from build123d import *

# Parameters (mm, degrees)
SKETCH2_R           = 2.75
BOSS_EXTRUDE1_DEPTH = 60
BOSS_EXTRUDE2_DEPTH = 2


with BuildPart() as part:
    # Sketch2 → Boss-Extrude1 (new body)
    with BuildSketch(Plane(origin=(0, 0, 0), x_dir=(1, 0, 0), z_dir=(0, 1, 0))):
        with BuildLine():
            Line((87, -11), (87, 88))
            ThreePointArc((87, 88), (84.656854249, 93.656854249), (79, 96))
            Line((79, 96), (39, 96))
            ThreePointArc((39, 96), (36.171572875, 94.828427125), (35, 92))
            Line((35, 92), (35, 44))
            ThreePointArc((35, 44), (33.828427125, 41.171572875), (31, 40))
            Line((31, 40), (-31, 40))
            ThreePointArc((-31, 40), (-33.828427125, 41.171572875), (-35, 44))
            Line((-35, 44), (-35, 92))
            ThreePointArc((-35, 92), (-36.171572875, 94.828427125), (-39, 96))
            Line((-39, 96), (-79, 96))
            ThreePointArc((-79, 96), (-84.656854249, 93.656854249), (-87, 88))
            Line((-87, 88), (-87, -11))
            ThreePointArc((-87, -11), (-84.656854249, -16.656854249), (-79, -19))
            Line((-79, -19), (-32, -19))
            ThreePointArc((-32, -19), (-29.171572875, -17.828427125), (-28, -15))
            Line((-28, -15), (-28, -3))
            ThreePointArc((-28, -3), (0, 25), (28, -3))
            Line((28, -3), (28, -15))
            ThreePointArc((28, -15), (29.171572875, -17.828427125), (32, -19))
            Line((32, -19), (79, -19))
            ThreePointArc((79, -19), (84.656854249, -16.656854249), (87, -11))
        make_face()
        with Locations(Location((-79, 88, 0), (0, 0, 270))):
            Circle(SKETCH2_R, mode=Mode.SUBTRACT)
        with Locations(Location((79, 88, 0), (0, 0, 270))):
            Circle(SKETCH2_R, mode=Mode.SUBTRACT)
        with Locations(Location((79, -11, 0), (0, 0, 270))):
            Circle(SKETCH2_R, mode=Mode.SUBTRACT)
        with Locations(Location((-79, -11, 0), (0, 0, 270))):
            Circle(SKETCH2_R, mode=Mode.SUBTRACT)
        with Locations(Location((0, 32.5, 0), (0, 0, 270))):
            Circle(SKETCH2_R, mode=Mode.SUBTRACT)
        with BuildLine():
            Line((-39, 93.5), (-71.5, 93.5))
            ThreePointArc((-71.5, 93.5), (-72.914213562, 92.914213562), (-73.5, 91.5))
            Line((-73.5, 91.5), (-73.5, 88))
            ThreePointArc((-73.5, 88), (-75.110912703, 84.110912703), (-79, 82.5))
            Line((-79, 82.5), (-82.5, 82.5))
            ThreePointArc((-82.5, 82.5), (-83.914213562, 81.914213562), (-84.5, 80.5))
            Line((-84.5, 80.5), (-84.5, -3.5))
            ThreePointArc((-84.5, -3.5), (-83.914213562, -4.914213562), (-82.5, -5.5))
            Line((-82.5, -5.5), (-79, -5.5))
            ThreePointArc((-79, -5.5), (-75.110912703, -7.110912703), (-73.5, -11))
            Line((-73.5, -11), (-73.5, -14.5))
            ThreePointArc((-73.5, -14.5), (-72.914213562, -15.914213562), (-71.5, -16.5))
            Line((-71.5, -16.5), (-32, -16.5))
            ThreePointArc((-32, -16.5), (-30.939339828, -16.060660172), (-30.5, -15))
            Line((-30.5, -15), (-30.5, -3))
            ThreePointArc((-30.5, -3), (-23.549354883, 16.382411734), (-5.865384615, 26.930707698))
            ThreePointArc((-5.865384615, 26.930707698), (-4.705780008, 27.622399237), (-4.25, 28.893377055))
            Line((-4.25, 28.893377055), (-4.25, 35.5))
            ThreePointArc((-4.25, 35.5), (-4.835786438, 36.914213562), (-6.25, 37.5))
            Line((-6.25, 37.5), (-31, 37.5))
            ThreePointArc((-31, 37.5), (-35.596194078, 39.403805922), (-37.5, 44))
            Line((-37.5, 44), (-37.5, 92))
            ThreePointArc((-37.5, 92), (-37.939339828, 93.060660172), (-39, 93.5))
        make_face(mode=Mode.SUBTRACT)
        with BuildLine():
            Line((30.5, -15), (30.5, -3))
            ThreePointArc((30.5, -3), (23.549354883, 16.382411734), (5.865384615, 26.930707698))
            ThreePointArc((5.865384615, 26.930707698), (4.705780008, 27.622399237), (4.25, 28.893377055))
            Line((4.25, 28.893377055), (4.25, 35.5))
            ThreePointArc((4.25, 35.5), (4.835786438, 36.914213562), (6.25, 37.5))
            Line((6.25, 37.5), (31, 37.5))
            ThreePointArc((31, 37.5), (35.596194078, 39.403805922), (37.5, 44))
            Line((37.5, 44), (37.5, 92))
            ThreePointArc((37.5, 92), (37.939339828, 93.060660172), (39, 93.5))
            Line((39, 93.5), (71.5, 93.5))
            ThreePointArc((71.5, 93.5), (72.914213562, 92.914213562), (73.5, 91.5))
            Line((73.5, 91.5), (73.5, 88))
            ThreePointArc((73.5, 88), (75.110912703, 84.110912703), (79, 82.5))
            Line((79, 82.5), (82.5, 82.5))
            ThreePointArc((82.5, 82.5), (83.914213562, 81.914213562), (84.5, 80.5))
            Line((84.5, 80.5), (84.5, -3.5))
            ThreePointArc((84.5, -3.5), (83.914213562, -4.914213562), (82.5, -5.5))
            Line((82.5, -5.5), (79, -5.5))
            ThreePointArc((79, -5.5), (75.110912703, -7.110912703), (73.5, -11))
            Line((73.5, -11), (73.5, -14.5))
            ThreePointArc((73.5, -14.5), (72.914213562, -15.914213562), (71.5, -16.5))
            Line((71.5, -16.5), (32, -16.5))
            ThreePointArc((32, -16.5), (30.939339828, -16.060660172), (30.5, -15))
        make_face(mode=Mode.SUBTRACT)
    extrude(amount=BOSS_EXTRUDE1_DEPTH)

    # Sketch3 → Boss-Extrude2 (add)
    # profile 1 of 2: a face of its own
    with BuildSketch(Plane.XZ):
        with BuildLine():
            Line((-37.5, -92), (-37.5, -44))
            ThreePointArc((-37.5, -44), (-35.596194078, -39.403805922), (-31, -37.5))
            Line((-31, -37.5), (-6.25, -37.5))
            ThreePointArc((-6.25, -37.5), (-4.835786438, -36.914213562), (-4.25, -35.5))
            Line((-4.25, -35.5), (-4.25, -28.893377055))
            ThreePointArc((-4.25, -28.893377055), (-4.705780008, -27.622399237), (-5.865384615, -26.930707698))
            ThreePointArc((-5.865384615, -26.930707698), (-23.549354883, -16.382411734), (-30.5, 3))
            Line((-30.5, 3), (-30.5, 15))
            ThreePointArc((-30.5, 15), (-30.939339828, 16.060660172), (-32, 16.5))
            Line((-32, 16.5), (-71.5, 16.5))
            ThreePointArc((-71.5, 16.5), (-72.914213562, 15.914213562), (-73.5, 14.5))
            Line((-73.5, 14.5), (-73.5, 11))
            ThreePointArc((-73.5, 11), (-75.110912703, 7.110912703), (-79, 5.5))
            Line((-79, 5.5), (-82.5, 5.5))
            ThreePointArc((-82.5, 5.5), (-83.914213562, 4.914213562), (-84.5, 3.5))
            Line((-84.5, 3.5), (-84.5, -80.5))
            ThreePointArc((-84.5, -80.5), (-83.914213562, -81.914213562), (-82.5, -82.5))
            Line((-82.5, -82.5), (-79, -82.5))
            ThreePointArc((-79, -82.5), (-75.110912703, -84.110912703), (-73.5, -88))
            Line((-73.5, -88), (-73.5, -91.5))
            ThreePointArc((-73.5, -91.5), (-72.914213562, -92.914213562), (-71.5, -93.5))
            Line((-71.5, -93.5), (-39, -93.5))
            ThreePointArc((-39, -93.5), (-37.939339828, -93.060660172), (-37.5, -92))
        make_face()
        with BuildLine():
            Line((-39.5, -91.5), (-39.5, -44))
            ThreePointArc((-39.5, -44), (-37.01040764, -37.98959236), (-31, -35.5))
            Line((-31, -35.5), (-6.25, -35.5))
            Line((-6.25, -35.5), (-6.25, -28.893377055))
            ThreePointArc((-6.25, -28.893377055), (-25.093574875, -17.653389552), (-32.5, 3))
            Line((-32.5, 3), (-32.5, 14.5))
            Line((-32.5, 14.5), (-71.5, 14.5))
            Line((-71.5, 14.5), (-71.5, 11))
            ThreePointArc((-71.5, 11), (-73.696699141, 5.696699141), (-79, 3.5))
            Line((-79, 3.5), (-82.5, 3.5))
            Line((-82.5, 3.5), (-82.5, -80.5))
            Line((-82.5, -80.5), (-79, -80.5))
            ThreePointArc((-79, -80.5), (-73.696699141, -82.696699141), (-71.5, -88))
            Line((-71.5, -88), (-71.5, -91.5))
            Line((-71.5, -91.5), (-39.5, -91.5))
        make_face(mode=Mode.SUBTRACT)
    # profile 2 of 2: a face of its own
    with BuildSketch(Plane.XZ):
        with BuildLine():
            Line((30.5, 15), (30.5, 3))
            ThreePointArc((30.5, 3), (23.549354883, -16.382411734), (5.865384615, -26.930707698))
            ThreePointArc((5.865384615, -26.930707698), (4.705780008, -27.622399237), (4.25, -28.893377055))
            Line((4.25, -28.893377055), (4.25, -35.5))
            ThreePointArc((4.25, -35.5), (4.835786438, -36.914213562), (6.25, -37.5))
            Line((6.25, -37.5), (31, -37.5))
            ThreePointArc((31, -37.5), (35.596194078, -39.403805922), (37.5, -44))
            Line((37.5, -44), (37.5, -92))
            ThreePointArc((37.5, -92), (37.939339828, -93.060660172), (39, -93.5))
            Line((39, -93.5), (71.5, -93.5))
            ThreePointArc((71.5, -93.5), (72.914213562, -92.914213562), (73.5, -91.5))
            Line((73.5, -91.5), (73.5, -88))
            ThreePointArc((73.5, -88), (75.110912703, -84.110912703), (79, -82.5))
            Line((79, -82.5), (82.5, -82.5))
            ThreePointArc((82.5, -82.5), (83.914213562, -81.914213562), (84.5, -80.5))
            Line((84.5, -80.5), (84.5, 3.5))
            ThreePointArc((84.5, 3.5), (83.914213562, 4.914213562), (82.5, 5.5))
            Line((82.5, 5.5), (79, 5.5))
            ThreePointArc((79, 5.5), (75.110912703, 7.110912703), (73.5, 11))
            Line((73.5, 11), (73.5, 14.5))
            ThreePointArc((73.5, 14.5), (72.914213562, 15.914213562), (71.5, 16.5))
            Line((71.5, 16.5), (32, 16.5))
            ThreePointArc((32, 16.5), (30.939339828, 16.060660172), (30.5, 15))
        make_face()
        with BuildLine():
            Line((71.5, 14.5), (32.5, 14.5))
            Line((32.5, 14.5), (32.5, 3))
            ThreePointArc((32.5, 3), (25.093574875, -17.653389552), (6.25, -28.893377055))
            Line((6.25, -28.893377055), (6.25, -35.5))
            Line((6.25, -35.5), (31, -35.5))
            ThreePointArc((31, -35.5), (37.01040764, -37.98959236), (39.5, -44))
            Line((39.5, -44), (39.5, -91.5))
            Line((39.5, -91.5), (71.5, -91.5))
            Line((71.5, -91.5), (71.5, -88))
            ThreePointArc((71.5, -88), (73.696699141, -82.696699141), (79, -80.5))
            Line((79, -80.5), (82.5, -80.5))
            Line((82.5, -80.5), (82.5, 3.5))
            Line((82.5, 3.5), (79, 3.5))
            ThreePointArc((79, 3.5), (73.696699141, 5.696699141), (71.5, 11))
            Line((71.5, 11), (71.5, 14.5))
        make_face(mode=Mode.SUBTRACT)
    extrude(amount=-BOSS_EXTRUDE2_DEPTH)


solid = part.part
The model under review builds one solid part; all positions refer to its coordinate system, in mm. A direction names the side the tool comes from. Coordinates: 2 decimals unless noted, no trailing zeros. Loops run counter-clockwise (first coordinate to the right, second up) from the corner with the lowest first, then second, coordinate; pieces in that order, holes last.
(1) Draft analysis for pull direction Z (two halves, no side actions). For faces 1 (the cylindrical face through (36.203, 29.58, -94.859)), 2 (the cylindrical face through (29.141, 29.58, 17.797)), 3 (the cylindrical face through (-23.7, 30.6, -16.2)), 4 (the flat face through (-87, 30, -39)), state which applies: +Z half, -Z half, draft (parallel to the pull), parting line (faces both ways), or undercut.
Determined:
face 1: -Z half
face 2: +Z half
face 3: undercut
face 4: draft
(2) Consider section B-B, the plane z = -58. Give the boundary of the cut face in (x, y), plus the area to 3 significant figures.
Determined:
outline: (-87, 0) - (-82.5, 0) - (-82.5, 2) - (-84.5, 2) - (-84.5, 60) - (-87, 60) - close; (-39.5, 0) - (-35, 0) - (-35, 60) - (-37.5, 60) - (-37.5, 2) - (-39.5, 2) - close; (35, 0) - (39.5, 0) - (39.5, 2) - (37.5, 2) - (37.5, 60) - (35, 60) - close; (82.5, 0) - (87, 0) - (87, 60) - (84.5, 60) - (84.5, 2) - (82.5, 2) - close
area: 616 mm2
(3) Tool access review of faces 5 (the cylindrical face through (73.755, 0.986, 5.639)), 6 (the flat face through (-28, 30, 9)), 7 (the flat face through (-84.5, 31, -39)), 8 (the cylindrical face through (-33.797, 29.58, -41.141)): name each direction out of +Z, -Z, +X, -X, +Y, -Y from which nothing blocks a thin tool from reaching the whole face with its end or side.
Determined:
face 5: +Y, -Y
face 6: +Z, +Y, -Y
face 7: +Y
face 8: -Z, +Y, -Y
(4) Consider section C-C, the plane y = 28. Give the number of separate pieces and of enclosed holes in the cut face, plus the area to 3 significant figures.
Determined:
separate pieces: 1
enclosed holes: 7
area: 2,210 mm2
(5) Consider section D-D, the plane z = -19. Give the boundary of the cut face in (x, y).
Determined:
outline: (-87, 0) - (-82.5, 0) - (-82.5, 2) - (-84.5, 2) - (-84.5, 60) - (-87, 60) - close; (-23.92, 0) - (-17.32, 0) - (-17.32, 60) - (-21.12, 60) - (-21.12, 2) - (-23.92, 2) - close; (17.32, 0) - (23.92, 0) - (23.92, 2) - (21.12, 2) - (21.12, 60) - (17.32, 60) - close; (82.5, 0) - (87, 0) - (87, 60) - (84.5, 60) - (84.5, 2) - (82.5, 2) - close
(6) Insertion check: P1, Ø1, axis at y = 33.5, z = 12, coming from the +X side; P2, Ø5, axis at x = 0, z = -32.5, coming from the -Y side; P3, Ø0.6, axis at y = 0.5, z = 12.5, coming from the -X side; P4, Ø2, axis at x = 4, y = 21, coming from the -Z side. Each pin has a flat end and moves straight along its axis. Give the tip position at first contact, or say it passes through.
Determined:
P1: stops at x = 86.98
P2: passes through
P3: stops at x = -86.91
P4: stops at z = -40
(7) Consider section A-A, the plane x = 65. Give the boundary of the cut face in (y, z), plus the area to 3 significant figures.
Determined:
outline: (0, -96) - (60, -96) - (60, -93.5) - (2, -93.5) - (2, -91.5) - (0, -91.5) - close; (0, 14.5) - (2, 14.5) - (2, 16.5) - (60, 16.5) - (60, 19) - (0, 19) - close
area: 308 mm2
(8) Wall thickness on L1, parallel to X at y = 41, z = -46; L2, parallel to X at y = 16.5, z = -88; L3, parallel to X at y = 30, z = 11: over which ranges is each line inside the solid? List them lowest first.
Determined:
L1: x = -87 to -84.5, -37.5 to -35, 35 to 37.5, 84.5 to 87
L2: x = -87 to -81.75, -76.25 to -73.5, -37.5 to -35, 35 to 37.5, 73.5 to 76.25, 81.75 to 87
L3: x = -87 to -81.75, -76.25 to -73.5, -30.5 to -28, 28 to 30.5, 73.5 to 76.25, 81.75 to 87
